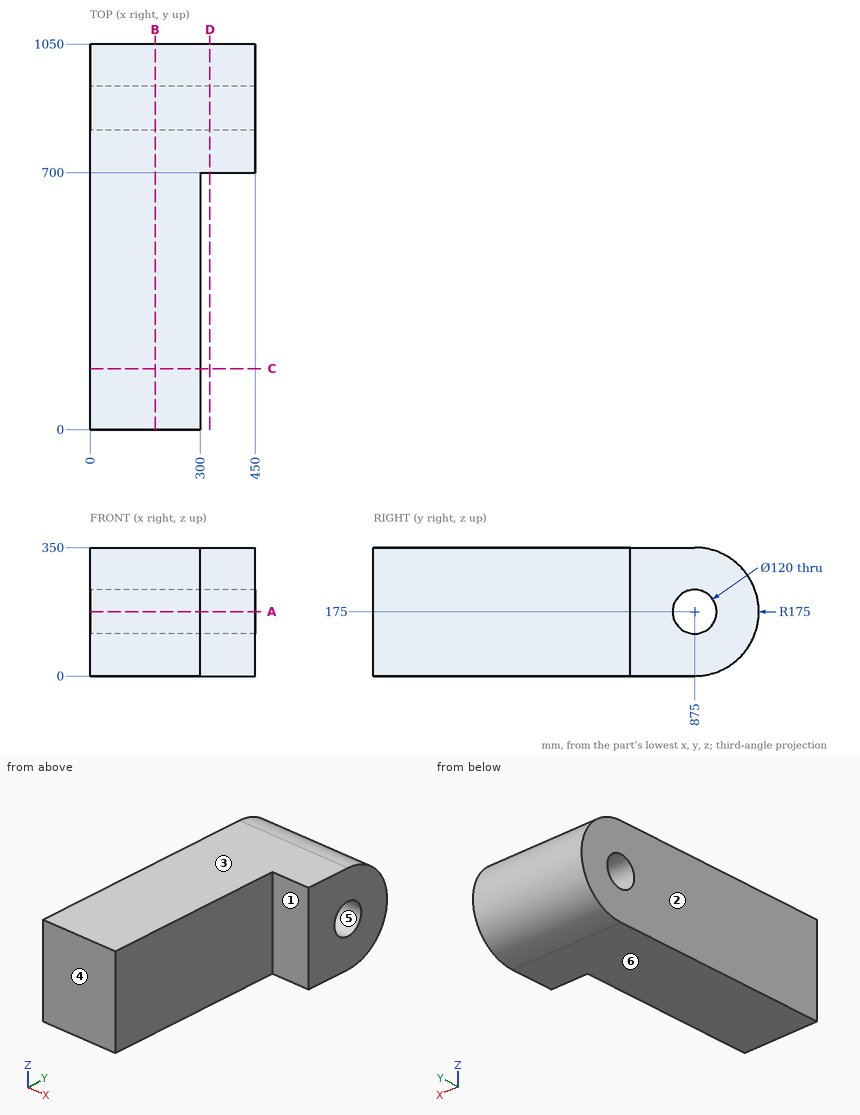
The figure shows three views and two pictorial views of one solid part (mm, origin at its lowest corner). Answer the questions. A direction names the side the tool comes from. Coordinates: 2 decimals unless noted, no trailing zeros. Loops run counter-clockwise (first coordinate to the right, second up) from the corner with the lowest first, then second, coordinate; pieces in that order, holes last. Notation, with made-up numbers: (18.25, 31) -> (39.25, 31) arc R34 cw to (39.25, 66) -> close; hole circle Ø3 at (25, 45.5). An arc over 180 degrees is marked (long way). Write item = value, one per line. Start each with the question number.
1) A cutting plane is placed at D-D (x = 326). Give the vertices of the cut face in (y, z), then the cut area to 3 significant figures.
2) A cutting plane is placed at B-B (x = 177). Give the vertices of the cut face in (y, z).
3) A cutting plane is placed at A-A (z = 175). Give the vertices of the cut face in (x, y).
4) A cutting plane is placed at C-C (y = 165.5). Give the vertices of the cut face in (x, z), then the cut area to 3 significant figures.
5) Straight lines are drawn through the part: line 1 (Y direction, x = 168, z = 175); line 2 (Y direction, x = 301, z = 175); line 3 (X direction, y = 310, z = 30.5). For each, find the intervals that lie inside material, in ascending order. Write a range as from..to.
6) Given pin 1 Ø1.5 at (x, y) = (86.5, 851) entering from -Z; pin 2 Ø5 at (x, z) = (364, 289) entering from +Y; pin 3 Ø10 at (x, z) = (60, 96) entering from +Y, each flat-ended and moving along its own axis, determine where each tip first touches the part or whether it passes through.
7) A tool of negligible diameter and unlimited length cuts with its end or side. For the marked faces 1 and 2, from which of +Z, -Z, +X, -X, +Y, -Y can it reach the whole face along a straight path? Write none if from no direction.
8) The mould has two halves that part along Z. Classify the marked faces 3, 4, 5 and 6: released by +Z, released by -Z, zero draft, split by the parting line, or undercut.
Responses:
q1.outline = (700, 0) -> (875, 0) arc R175 ccw to (875, 350) -> (700, 350) -> close; hole circle Ø120 at (875, 175)
q1.area = 98,000 mm²
q2.outline = (0, 0) -> (875, 0) arc R175 ccw to (875, 350) -> (0, 350) -> close; hole circle Ø120 at (875, 175)
q3.outline = (0, 0) -> (300, 0) -> (300, 700) -> (450, 700) -> (450, 815) -> (0, 815) -> close; (0, 935) -> (450, 935) -> (450, 1050) -> (0, 1050) -> close
q4.outline = (0, 0) -> (300, 0) -> (300, 350) -> (0, 350) -> close
q4.area = 105,000 mm²
q5.line_1 = 0..815, 935..1050
q5.line_2 = 700..815, 935..1050
q5.line_3 = 0..300
q6.pin_1 = 0
q6.pin_2 = 1009.88
q6.pin_3 = 1033.58
q7.face_1 = +Z, -Z, +X, -Y
q7.face_2 = +Z, -Z, -X, +Y, -Y
q8.face_3 = released by +Z
q8.face_4 = zero draft
q8.face_5 = undercut
q8.face_6 = released by -Z
